For this review, take the finished solid that the model builds, in its own axes (mm). Face numbers are marked on the shaded views. A direction names the side the tool comes from. Round coordinates to 2 decimals unless told otherwise and drop trailing zeros. Write each loop counter-clockwise with the first axis right and the second up, starting at its lowest first coordinate (ties: lowest second). Pieces come first, ordered by that corner, then holes. Notation, with made-up numbers: (18, 73) -> (55, 73) arc R37 ccw to (55, 109) -> close; hole circle Ø1 at (63.25, -2). An arc over 180 degrees is marked (long way). Answer as CSV lines item,"result". Start each with the question number.
Item 1: Mouldability with a two-part tool opening along X and no side actions: class the marked faces 1, 2, 3 and 4 as +X half, -X half, draft (parallel to the pull), parting line (faces both ways), or undercut.
Item 2: Take a section at C-C on x = -56.5. Give the boundary of the cut face in (y, z), then the cut area to 3 significant figures.
Item 3: Machinability: for the marked faces 5, 6, 7 and 8, which of the approach directions +Z, -Z, +X, -X, +Y, -Y give a long, thin tool a straight path to every point of the face, cutting with its end or side? Answer none if there is none.
Item 4: Wall thickness on probe 1 along X at (y, z) = (-7.5, 10.5); probe 2 along X at (y, z) = (-14, -10); probe 3 along X at (y, z) = (-10.5, 7.5): over which ranges is each line inside the solid? List them lowest first. Write a range as from..to.
Item 5: Take a section at A-A on z = 4.5. Give the boundary of the cut face in (x, y).
Item 6: For pin 1 Ø8 at (x, z) = (20.5, 0.5) entering from +Y; pin 2 Ø10 at (x, z) = (-56.5, -9.5) entering from -Y; pin 3 Ø1.8 at (x, z) = (-69, -4.5) entering from -Y, all flat-tipped, find the tip position at first contact; note any pin that passes through.
Item 7: Take a section at B-B on y = -14.75. Give the boundary of the cut face in (x, z).
```python
from build123d import *

# Parameters (mm, degrees)
SKETCH_5_W        = 6
SKETCH_5_H        = 30
EXTRUDE_2_DEPTH   = 10
EXTRUDE_2_2_DEPTH = 10
SKETCH_6_W        = 6
SKETCH_6_H        = 30
EXTRUDE_3_DEPTH   = 10
EXTRUDE_4_DEPTH   = 3
EXTRUDE_5_DEPTH   = 127


with BuildPart() as part:
    # Sketch 5 → Extrude 2 (new body)
    with BuildSketch(Plane(origin=(0, 0, 0), x_dir=(1, 0, 0), z_dir=(0, 1, 0))):
        with Locations((68, 0)):
            Rectangle(SKETCH_5_W, SKETCH_5_H)
    extrude(amount=-EXTRUDE_2_DEPTH)

    # Sketch 6 → Extrude 3 (add)
    with BuildSketch(Plane.XZ.offset(10)):
        with Locations((68, 0)):
            Rectangle(SKETCH_6_W, SKETCH_6_H)
    extrude(amount=EXTRUDE_3_DEPTH)



with BuildPart() as body_2:
    # Sketch 5 → Extrude 2 2 (new body)
    with BuildSketch(Plane(origin=(0, 0, 0), x_dir=(1, 0, 0), z_dir=(0, 1, 0))):
        with Locations((-68, 0)):
            Rectangle(SKETCH_5_W, SKETCH_5_H)
    extrude(amount=-EXTRUDE_2_2_DEPTH)

    # Sketch 8 → Extrude 4 (add)
    with BuildSketch(Plane(origin=(-65, 0, 0), x_dir=(0, 0, -1), z_dir=(1, 0, 0))):
        Polygon((15, -14), (15, -20), (-15, -20), (-15, 0), (15, 0), align=None)
    extrude(amount=EXTRUDE_4_DEPTH)


with BuildPart() as part_1:
    add(part.part)

    add(body_2.part)  # Extrude 5 merges body 2
    # Sketch 7 → Extrude 5 (add)
    with BuildSketch(Plane.ZY.offset(-65)):
        Polygon((-15, -17), (-15, -20), (15, -9), (15, -6), align=None)
    extrude(amount=EXTRUDE_5_DEPTH)


solid = part_1.part
```
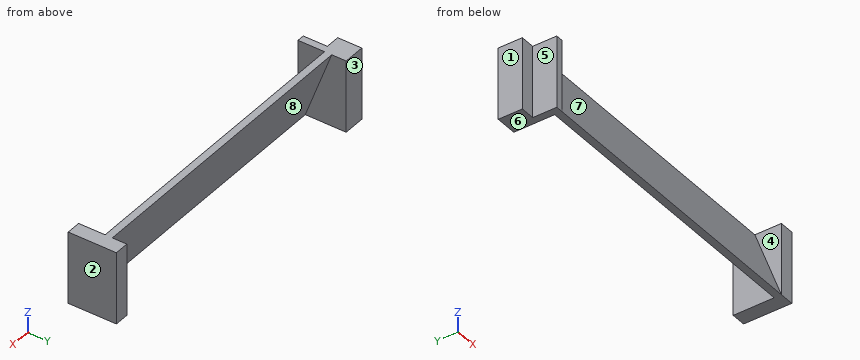
Output values:
1,face 1,"-X half"
1,face 2,"+X half"
1,face 3,"draft"
1,face 4,"undercut"
2,outline,"(-20, -15) -> (-17, -15) -> (-6, 15) -> (-9, 15) -> close"
2,area,"90.0 mm^2"
3,face 5,"+Z, -Z, -X, -Y"
3,face 6,"-Z, +X, -X, +Y, -Y"
3,face 7,"+Z, -Y"
3,face 8,"-Z, +Y"
4,probe 1,"x = -71..-62, 65..71"
4,probe 2,"x = -65..-62, 65..71"
4,probe 3,"x = -65..71"
5,outline,"(-71, -10) -> (-65, -10) -> (-65, -20) -> (-62, -20) -> (-62, -12.85) -> (65, -12.85) -> (65, -20) -> (71, -20) -> (71, 0) -> (65, 0) -> (65, -9.85) -> (-62, -9.85) -> (-62, 0) -> (-71, 0) -> close"
6,pin 1,"stops at y = -9.85"
6,pin 2,"stops at y = -19.82"
6,pin 3,"stops at y = -10"
7,outline,"(-65, -15) -> (-62, -15) -> (-62, -8.86) -> (65, -8.86) -> (65, -15) -> (71, -15) -> (71, 15) -> (65, 15) -> (65, -0.68) -> (-62, -0.68) -> (-62, 15) -> (-65, 15) -> close"
